Could you check a few things on this model? Use its own coordinates, in mm. Coordinates: 2 decimals unless noted, no trailing zeros. Write each loop counter-clockwise with the first axis right and the second up, starting at its lowest first coordinate (ties: lowest second). Pieces come first, ordered by that corner, then holes.
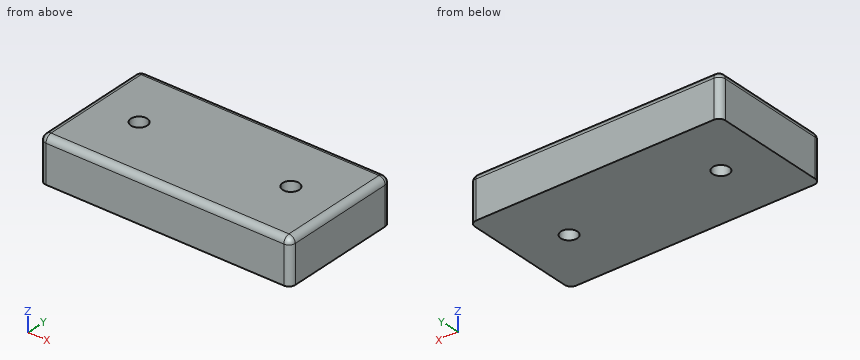
```python
from build123d import *

# Parameters (mm, degrees)
F0_W     = 39.6
F0_H     = 19.6
F0_R     = 1.3
F1_DEPTH = 7
F2_R     = 1


with BuildPart() as f1:
    # F0 (on Top) → F1 (new body)
    with BuildSketch(Plane.XY):
        Rectangle(F0_W, F0_H)
        with Locations((-12, 0)):
            Circle(F0_R, mode=Mode.SUBTRACT)
        with Locations((12, 0)):
            Circle(F0_R, mode=Mode.SUBTRACT)
    extrude(amount=F1_DEPTH)

    # F2
    f2_edges = [f1.edges().sort_by_distance(p)[0] for p in [
        (0, 9.8, 7),
        (19.8, 0, 7),
        (0, -9.8, 7),
        (19.8, 9.8, 3.5),
        (19.8, -9.8, 3.5),
        (-19.8, -9.8, 3.5),
        (-19.8, 9.8, 3.5),
        (-19.8, 0, 7),
    ]]
    fillet(f2_edges, radius=F2_R)


solid = f1.part
```
Item 1: I want a section at A-A, the plane x = 12. List the corners of the cut face in (y, z) for me.
Item 2: If I drill on line 1 along Y through (x, z) = (12, 2.75); line 2 along X through (y, z) = (0.5, 6.25); line 3 along X through (y, z) = (-6.5, 6.5), over which ranges is the centre line in solid material (lowest first)?
Item 3: I want a section at B-B, the plane y = 0. List the corners of the cut face in (x, z) for me, then the cut area to 3 significant figures.
Item 4: Will this pin go through, and if not, where does the flat tip stop? pin 1 Ø1.6 at (x, y) = (12, 0) entering from +Z.
Taken from the geometry:
1. outline: (-9.8, 0) - (-1.3, 0) - (-1.3, 7) - (-8.8, 7) arc R1 ccw to (-9.8, 6) - close; (1.3, 0) - (9.8, 0) - (9.8, 6) arc R1 ccw to (8.8, 7) - (1.3, 7) - close
2. line 1: y = -9.8 to -1.3, 1.3 to 9.8
2. line 2: x = -19.77 to -13.2, -10.8 to 10.8, 13.2 to 19.77
2. line 3: x = -19.67 to 19.67
3. outline: (-19.8, 0) - (-13.3, 0) - (-13.3, 7) - (-18.8, 7) arc R1 ccw to (-19.8, 6) - close; (-10.7, 0) - (10.7, 0) - (10.7, 7) - (-10.7, 7) - close; (13.3, 0) - (19.8, 0) - (19.8, 6) arc R1 ccw to (18.8, 7) - (13.3, 7) - close
3. area: 240 mm2
4. pin 1: passes through
